Input: part model. Units: mm. Frame: model coordinates. A direction names the side the tool comes from. Coordinates: 2 decimals unless noted, no trailing zeros. Write each loop counter-clockwise with the first axis right and the second up, starting at its lowest first coordinate (ties: lowest second). Pieces come first, ordered by that corner, then holes. Notation, with made-up numbers: (70.5, 77.25) - (108.5, 77.25) arc R11 cw to (108.5, 93.25) - close; hole circle Ø7 at (42, -40). An arc over 180 degrees is marked (long way). Put each result on its own line as item: value. Start each with the question number.
1. Pin query (flat end, axial travel): pin 1 (1.3 mm diameter, centred on y = 0, z = -6.35, fed in from -X); pin 2 (10 mm diameter, centred on x = 186, z = 11.5, fed in from +Y); pin 3 (1.9 mm diameter, centred on y = 0, z = -6.35, fed in from +X); pin 4 (8 mm diameter, centred on x = 33, z = 13, fed in from -Y). Return the tip coordinate at first contact, or that it passes through.
2. Cut plane A-A, the plane x = 178.5. Return loops of the section in (y, z), and give its area (3 significant figures).
3. Cut plane B-B, the plane x = 45.5. Return loops of the section in (y, z).
4. Pull-direction query (X, two-part tool) for faces 1 (the conical face through (137.427, -11.672, -8.95)), 2 (the conical face through (222.38, 8.6, 0.24)), 3 (the cylindrical face through (207.72, -13.22, -10.14)); classes: released by +X, released by -X, zero draft, split by the parting line, or undercut.
5. Access query for faces 4 (the flat face through (257.81, 0, -3)), 5 (the conical face through (187.39, -3.69, -7.77)), 6 (the cylindrical face through (66.14, -2.75, -12.4)), 7 (the cylindrical face through (190.325, 13.311, -0.553)). Directions: +Z, -Z, +X, -X, +Y, -Y. A direction counts if a zero-diameter tool reaches every point of the face in a straight line with its end or side. Return the directions, or none.
6. Line query: line 1 (Z direction, x = 101.5, y = 0); line 2 (Y direction, x = 25, z = 0.5); line 3 (Y direction, x = 255.25, z = 6.35). Output: solid intervals per line, ascending.
from build123d import *

# Parameters (mm, degrees)
SKETCH3_R                             = 0.79375
CUT_EXTRUDE1_DEPTH                    = 258.810003035
SKETCH4_R                             = 1.5875
CUT_EXTRUDE2_DEPTH                    = 12.7
TAP_DRILL_FOR_10_HELICOIL2_AT_2_COUNT = 2
TAP_DRILL_FOR_10_HELICOIL2_AT_2_PITCH = 34.925
CIRPATTERN2_COUNT                     = 3
CIRPATTERN2_ANGLE                     = 230
SKETCH11_R                            = 1.5875
CUT_EXTRUDE3_DEPTH                    = 12.7


with BuildPart() as part:
    # Sketch1 → Revolve1 (revolve)
    with BuildSketch(Plane.XY):
        with BuildLine():
            Line((12.7, 12.7), (118.11, 12.7))
            Line((118.11, 12.7), (156.210003035, 16.662289952))
            Line((156.210003035, 16.662289952), (257.810003035, 16.662289952))
            Line((257.810003035, 16.662289952), (257.810003035, 0))
            Line((257.810003035, 0), (0, 0))
            ThreePointArc((0, 0), (3.719743879, 8.980256121), (12.7, 12.7))
        make_face()
    revolve(axis=Axis((0, 0, 0), (1, 0, 0)))

    # Sketch3 → Cut-Extrude1 (cut, through all)
    with BuildSketch(Plane(origin=(257.810003035, 0, 0), x_dir=(0, 0, -1), z_dir=(1, 0, 0))):
        Circle(SKETCH3_R)
        with Locations((6.35, 0)):
            Circle(SKETCH3_R)
        with Locations((-6.35, 0)):
            Circle(SKETCH3_R)
        with Locations((0, 6.35)):
            Circle(SKETCH3_R)
        with Locations((0, -6.35)):
            Circle(SKETCH3_R)
    extrude(amount=-CUT_EXTRUDE1_DEPTH, mode=Mode.SUBTRACT)

    # Sketch4 → Cut-Extrude2 (cut)
    with BuildSketch(Plane(origin=(257.810003035, 0, 0), x_dir=(0, 0, -1), z_dir=(1, 0, 0))):
        with Locations((-6.35, 0)):
            Circle(SKETCH4_R)
        with Locations((6.35, 0)):
            Circle(SKETCH4_R)
    extrude(amount=-CUT_EXTRUDE2_DEPTH, mode=Mode.SUBTRACT)

    # Sketch8 → Tap Drill for #10 Helicoil2 (revolve, cut)
    with BuildSketch(Plane(origin=(222.758003035, 16.662289952, 0), x_dir=(0, 0, 1), z_dir=(1, 0, 0))):
        Polygon((0, 0), (0, 8.3312), (2.5527, 6.797383098), (2.5527, 0), align=None)
    tap_drill_for_10_helicoil2 = revolve(axis=Axis((222.758003035, 23.012289952, 0), (0, -1, 0)), mode=Mode.SUBTRACT)

    # Tap Drill for #10 Helicoil2 at 2: Tap Drill for #10 Helicoil2 ×2
    with Locations(*[(-i * TAP_DRILL_FOR_10_HELICOIL2_AT_2_PITCH, 0, 0) for i in range(1, TAP_DRILL_FOR_10_HELICOIL2_AT_2_COUNT)]):
        add(tap_drill_for_10_helicoil2, mode=Mode.SUBTRACT)

    # CirPattern2: Tap Drill for #10 Helicoil2 ×3 about axis
    cirpattern2_axis = Axis((257.810003035, 0, 0), (-1, 0, 0))
    for i in range(1, CIRPATTERN2_COUNT):
        add(tap_drill_for_10_helicoil2.rotate(cirpattern2_axis, i * CIRPATTERN2_ANGLE / (CIRPATTERN2_COUNT - 1)), mode=Mode.SUBTRACT)

    # CirPattern2 copy 1 sketch → CirPattern2 copy 1 (revolve, cut)
    with BuildSketch(Plane(origin=(187.833003035, -7.041788016, -15.101163133), x_dir=(0, 0.906307787, -0.422618262), z_dir=(1, 0, 0))):
        Polygon((0, 0), (0, 8.3312), (2.5527, 6.797383098), (2.5527, 0), align=None)
    revolve(axis=Axis((187.833003035, -9.725413978, -20.856217581), (0, 0.422618262, 0.906307787)), mode=Mode.SUBTRACT)

    # CirPattern2 copy 2 sketch → CirPattern2 copy 2 (revolve, cut)
    with BuildSketch(Plane(origin=(187.833003035, -10.71031353, 12.764054627), x_dir=(0, -0.766044443, -0.64278761), z_dir=(1, 0, 0))):
        Polygon((0, 0), (0, 8.3312), (2.5527, 6.797383098), (2.5527, 0), align=None)
    revolve(axis=Axis((187.833003035, -14.792014851, 17.628436841), (0, 0.64278761, -0.766044443)), mode=Mode.SUBTRACT)

    # Sketch11 → Cut-Extrude3 (cut)
    with BuildSketch(Plane(origin=(257.810003035, 0, 0), x_dir=(0, 0, -1), z_dir=(1, 0, 0))):
        with Locations((-6.35, 6.35)):
            Circle(SKETCH11_R)
    extrude(amount=-CUT_EXTRUDE3_DEPTH, mode=Mode.SUBTRACT)


solid = part.part
Report:
1. pin 1: passes through
1. pin 2: stops at y = 15.34
1. pin 3: stops at x = 245.11
1. pin 4: stops at y = -8.96
2. outline: circle Ø33.32 at (0, 0); hole circle Ø1.59 at (-6.35, 0); hole circle Ø1.59 at (0, -6.35); hole circle Ø1.59 at (0, 0); hole circle Ø1.59 at (0, 6.35); hole circle Ø1.59 at (6.35, 0)
2. area: 862 mm^2
3. outline: circle Ø25.4 at (0, 0); hole circle Ø1.59 at (-6.35, 0); hole circle Ø1.59 at (0, -6.35); hole circle Ø1.59 at (0, 0); hole circle Ø1.59 at (0, 6.35); hole circle Ø1.59 at (6.35, 0)
4. face 1: released by -X
4. face 2: undercut
4. face 3: zero draft
5. face 4: +Z, -Z, +X, +Y, -Y
5. face 5: none
5. face 6: -X
5. face 7: +Y
6. line 1: z = -12.7 to -7.14, -5.56 to -0.79, 0.79 to 5.56, 7.14 to 12.7
6. line 2: y = -12.69 to -6.97, -5.73 to -0.62, 0.62 to 5.73, 6.97 to 12.69
6. line 3: y = -15.4 to -1.59, 1.59 to 4.76, 7.94 to 15.4
